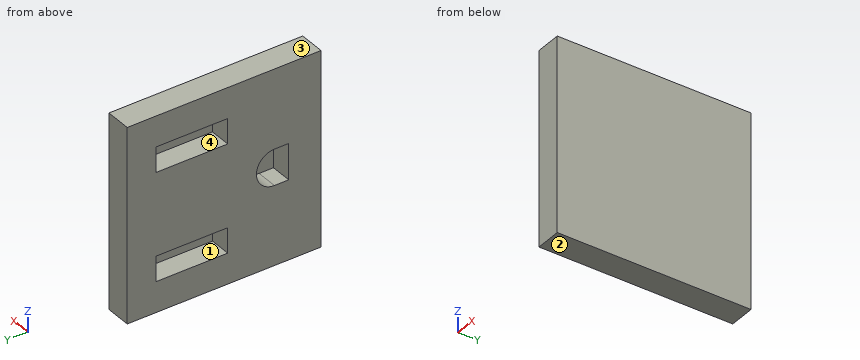
from build123d import *

# Parameters (mm, degrees)
SKETCH1_W           = 27
SKETCH1_H           = 27
BOSS_EXTRUDE1_DEPTH = 3.6
SKETCH2_W           = 3.5
SKETCH2_H           = 10
CUT_EXTRUDE1_DEPTH  = 3


with BuildPart() as part:
    # Sketch1 → Boss-Extrude1 (new body)
    with BuildSketch(Plane(origin=(0, 0, 0), x_dir=(0, 0, -1), z_dir=(1, 0, 0))):
        Rectangle(SKETCH1_W, SKETCH1_H)
    extrude(amount=BOSS_EXTRUDE1_DEPTH)

    # Sketch2 → Cut-Extrude1 (cut)
    with BuildSketch(Plane.ZY):
        with BuildLine():
            Line((-2.5, -7), (-2.5, -9))
            Line((-2.5, -9), (2.5, -9))
            Line((2.5, -9), (2.5, -7))
            ThreePointArc((2.5, -7), (0, -4.5), (-2.5, -7))
        make_face()
        with Locations((-7.5, 4.5)):
            Rectangle(SKETCH2_W, SKETCH2_H)
        with Locations((7.5, 4.5)):
            Rectangle(SKETCH2_W, SKETCH2_H)
    extrude(amount=-CUT_EXTRUDE1_DEPTH, mode=Mode.SUBTRACT)


solid = part.part
The model under review builds one solid part; all positions refer to its coordinate system, in mm. Face numbers are marked on the shaded views. Coordinates: 2 decimals unless noted, no trailing zeros. Loops run counter-clockwise (first coordinate to the right, second up) from the corner with the lowest first, then second, coordinate; pieces in that order, holes last. Notation, with made-up numbers: (47, 54.25) -> (97, 54.25) arc R24 cw to (97, 78.25) -> close; hole circle Ø7 at (-1.75, 86). An arc over 180 degrees is marked (long way). Use a Markdown table: item, result. Add a question column.
1. Add section C-C on z = -7. Write out the cut boundary in (x, y).
2. To check wall thickness, follow line 1 (Z direction, x = 2.35, y = 1.25); line 2 (Z direction, x = 2.75, y = -8.25); line 3 (Y direction, x = 2.1, z = 0). State the ranges of each line that lie inside material, in increasing order.
3. Clearance check with a flat-ended pin moving along its axis: pin 1 Ø1.8 at (y, z) = (5, 8) entering from -X. State where the tip first meets the part, or that it passes through.
4. Add section B-B on z = 0. Write out the cut boundary in (x, y).
5. Draft analysis for pull direction Z (two halves, no side actions). For the marked faces 1, 2, 3 and 4, state which applies: pulls with the +Z half, pulls with the -Z half, needs draft (parallel to the pull), parting line crosses it, or undercut.
6. Add section A-A on x = 0.35. Write out the cut boundary in (y, z).
Returned:
| question | item | result |
|---|---|---|
| 1 | outline | (0, -13.5) -> (3.6, -13.5) -> (3.6, 13.5) -> (0, 13.5) -> (0, 9.5) -> (3, 9.5) -> (3, -0.5) -> (0, -0.5) -> close |
| 2 | line 1 | z = -13.5 to -9.25, -5.75 to 5.75, 9.25 to 13.5 |
| 2 | line 2 | z = -13.5 to -2.5, 2.5 to 13.5 |
| 2 | line 3 | y = -13.5 to -9, -4.5 to 13.5 |
| 3 | pin 1 | stops at x = 3 |
| 4 | outline | (0, -13.5) -> (3.6, -13.5) -> (3.6, 13.5) -> (0, 13.5) -> (0, -4.5) -> (3, -4.5) -> (3, -9) -> (0, -9) -> close |
| 5 | face 1 | undercut |
| 5 | face 2 | pulls with the -Z half |
| 5 | face 3 | pulls with the +Z half |
| 5 | face 4 | undercut |
| 6 | outline | (-13.5, -13.5) -> (13.5, -13.5) -> (13.5, 13.5) -> (-13.5, 13.5) -> close; hole (-9, -2.5) -> (-7, -2.5) arc R2.5 ccw to (-7, 2.5) -> (-9, 2.5) -> close; hole (-0.5, -9.25) -> (9.5, -9.25) -> (9.5, -5.75) -> (-0.5, -5.75) -> close; hole (-0.5, 5.75) -> (9.5, 5.75) -> (9.5, 9.25) -> (-0.5, 9.25) -> close |
